```python
from build123d import *

# Parameters (mm, degrees)
BOSS_EXTRUDE1_DEPTH = 98.425
CUT_EXTRUDE1_REACH  = 692.094


with BuildPart() as part:
    # Sketch1 → Boss-Extrude1 (new body)
    with BuildSketch(Plane.XY):
        with BuildLine():
            Line((0, 35.8), (664.20000002, 35.8))
            ThreePointArc((664.20000002, 35.8), (682.10000002, 17.9), (664.20000002, 0))
            Line((664.20000002, 0), (0, 0))
            ThreePointArc((0, 0), (-17.9, 17.9), (0, 35.8))
        make_face()
    extrude(amount=BOSS_EXTRUDE1_DEPTH)

    # Sketch3 → Cut-Extrude1 (cut, up to next)
    with BuildSketch(Plane.XY.offset(98.425), mode=Mode.PRIVATE) as cut_extrude1_sk1:
        with BuildLine():
            Line((0, 34.1), (664.20000002, 34.1))
            ThreePointArc((664.20000002, 34.1), (680.40000002, 17.9), (664.20000002, 1.7))
            Line((664.20000002, 1.7), (0, 1.7))
            ThreePointArc((0, 1.7), (-16.2, 17.9), (0, 34.1))
        make_face()
    cut_extrude1_tool1 = extrude(cut_extrude1_sk1.sketch, amount=-CUT_EXTRUDE1_REACH, mode=Mode.PRIVATE) & part.part
    add(cut_extrude1_tool1.solids().sort_by_distance((332.1, 17.9, 98.425))[0], mode=Mode.SUBTRACT)


solid = part.part
```
The model under review builds one solid part; all positions refer to its coordinate system, in mm. A direction names the side the tool comes from. Round coordinates to 2 decimals unless told otherwise and drop trailing zeros. Write each loop counter-clockwise with the first axis right and the second up, starting at its lowest first coordinate (ties: lowest second). Pieces come first, ordered by that corner, then holes. Notation, with made-up numbers: (22.25, 24.5) -> (42.25, 24.5) arc R34 cw to (42.25, 62.5) -> close; hole circle Ø8 at (58, 14.25). An arc over 180 degrees is marked (long way). Use CSV: the item, a comma, the result in double quotes.
Q1. Mouldability with a two-part tool opening along X and no side actions: class faces 1 (the cylindrical face through (-16.196, 17.544, 49.901)), 2 (the flat face through (327, 34.1, 50)), 3 (the cylindrical face through (682.096, 18.294, 48.524)), 4 (the flat face through (327, 35.8, 49)) as released by +X, released by -X, zero draft, split by the parting line, or undercut.
Checks:
face 1,"undercut"
face 2,"undercut"
face 3,"released by +X"
face 4,"zero draft"
Q2. For pin 1 Ø5 at (y, z) = (23.5, 24.5) entering from -X; pin 2 Ø5 at (y, z) = (25.5, 82) entering from -X, all flat-tipped, find the tip position at first contact; note any pin that passes through.
Checks:
pin 1,"x = -17.63"
pin 2,"x = -17.16"
Q3. Consider section A-A (y = 17.9). Give the boundary of the cut face in (x, z) (3 decimals), then the cut area to 3 significant figures.
Checks:
outline,"(-17.9, 0) -> (-16.2, 0) -> (-16.2, 98.425) -> (-17.9, 98.425) -> close; (680.4, 0) -> (682.1, 0) -> (682.1, 98.425) -> (680.4, 98.425) -> close"
area,"335 mm²"
Q4. For faces 5 (the flat face through (337, 1.7, 50)), 6 (the flat face through (334, 35, 0)), list the 3-axis set-ups (+Z, -Z, +X, -X, +Y, -Y) from which the entire face can be reached by the end or side of a thin tool; tool diameter is ignored.
Checks:
face 5,"+Z, -Z"
face 6,"-Z, +X, -X, +Y, -Y"
Q5. To check wall thickness, follow probe 1 along Y at (x, z) = (636, 46); probe 2 along X at (y, z) = (17.5, 78.5); probe 3 along X at (y, z) = (23, 91). State the ranges of each line that lie inside material, in increasing order. Write a range as [from, to].
Checks:
probe 1,"[0, 1.7], [34.1, 35.8]"
probe 2,"[-17.9, -16.2], [680.4, 682.1]"
probe 3,"[-17.16, -15.38], [679.58, 681.36]"
Q6. Consider section B-B (x = 621). Give the boundary of the cut face in (y, z) (3 decimals).
Checks:
outline,"(0, 0) -> (1.7, 0) -> (1.7, 98.425) -> (0, 98.425) -> close; (34.1, 0) -> (35.8, 0) -> (35.8, 98.425) -> (34.1, 98.425) -> close"
Q7. Consider section C-C (z = 39.5). Give the boundary of the cut face in (x, y).
Checks:
outline,"(0, 0) -> (664.2, 0) arc R17.9 ccw to (664.2, 35.8) -> (0, 35.8) arc R17.9 ccw to start; hole (0, 1.7) -> (664.2, 1.7) arc R16.2 ccw to (664.2, 34.1) -> (0, 34.1) arc R16.2 ccw to start"
